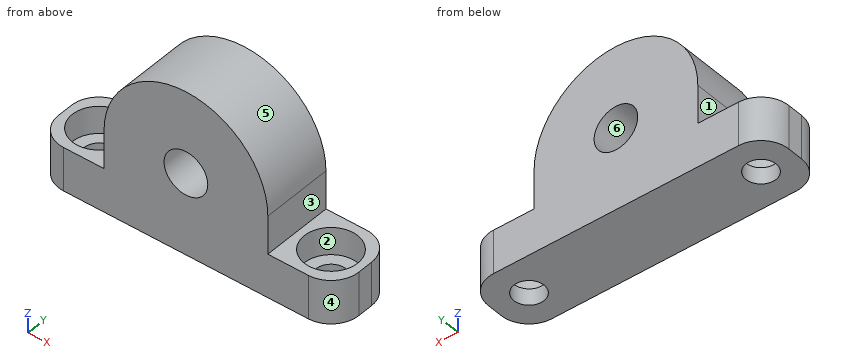
```python
from build123d import *

# Parameters (mm, degrees)
F0_R           = 4
F1_DEPTH       = 13
F3_D           = 5.5
F3_CBORE_D     = 9.75
F3_CBORE_DEPTH = 5
F4_R           = 5.08


with BuildPart() as f1:
    # F0 (on Front) → F1 (new body)
    with BuildSketch(Plane.XZ):
        with BuildLine():
            Line((-27.5, 8), (-27.5, 0))
            Line((-27.5, 0), (27.5, 0))
            Line((27.5, 0), (27.5, 8))
            Line((27.5, 8), (15, 8))
            Line((15, 8), (15, 15))
            ThreePointArc((15, 15), (0, 30), (-15, 15))
            Line((-15, 15), (-15, 8))
            Line((-15, 8), (-27.5, 8))
        make_face()
        with Locations((0, 15)):
            Circle(F0_R, mode=Mode.SUBTRACT)
    extrude(amount=F1_DEPTH)

    # F3 (through all)
    with Locations(Plane.XY.offset(8)):
        with Locations((-21.25, -6.5), (21.25, -6.5)):
            CounterBoreHole(F3_D / 2, F3_CBORE_D / 2, F3_CBORE_DEPTH)

    # F4
    f4_edges = [f1.edges().sort_by_distance(p)[0] for p in [
        (27.5, -13, 4),
        (27.5, 0, 4),
        (-27.5, -13, 4),
        (-27.5, 0, 4),
    ]]
    fillet(f4_edges, radius=F4_R)


solid = f1.part
```
Geometry: final body of the model. Coordinates: model frame, mm. Face numbers are marked on the shaded views. A direction names the side the tool comes from. Give positions to 0.01 mm unless a question says otherwise; leave off trailing zeros. Loops run counter-clockwise (first coordinate to the right, second up) from the corner with the lowest first, then second, coordinate; pieces in that order, holes last. Notation, with made-up numbers: (-11.75, 41) -> (28.25, 41) arc R21 ccw to (28.25, 69) -> close; hole circle Ø8 at (89.25, 38). An arc over 180 degrees is marked (long way). Return JSON: item names as keys, results as strings.
Item 1: Pin query (flat end, axial travel): P1, Ø4, axis at x = -16, y = -11, coming from the -Z side; P2, Ø3.5, axis at y = -9.5, z = 12.5, coming from the +X side; P3, Ø2, axis at x = -11.5, y = -7, coming from the +Z side; P4, Ø6, axis at x = -18.5, y = -5, coming from the +Z side. Return the tip coordinate at first contact, or that it passes through.
Filled in:
{"P1": "z = 0", "P2": "x = 15", "P3": "z = 25.71", "P4": "z = 8"}
Item 2: Line query: line 1 (Y direction, x = 21.25, z = 0.7); line 2 (Z direction, x = 0, y = -7); line 3 (Y direction, x = -21.25, z = 6.3) (3 decimals). Output: solid intervals per line, ascending.
Filled in:
{"line 1": "-13 to -9.25, -3.75 to 0", "line 2": "0 to 11, 19 to 30", "line 3": "-13 to -11.375, -1.625 to 0"}
Item 3: Section D-D, the plane y = -10.5. Output: boundary loops of the cut face in (x, z), plus the area to 3 significant figures.
Filled in:
{"outline": "(-26.8, 0) -> (26.8, 0) -> (26.8, 8) -> (24.04, 8) -> (24.04, 3) -> (18.46, 3) -> (18.46, 8) -> (15, 8) -> (15, 15) arc R15 ccw to (-15, 15) -> (-15, 8) -> (-18.46, 8) -> (-18.46, 3) -> (-24.04, 3) -> (-24.04, 8) -> (-26.8, 8) -> close; hole circle Ø8 at (0, 15)", "area": "886 mm^2"}
Item 4: Access query for the marked faces 1, 2 and 3. Directions: +Z, -Z, +X, -X, +Y, -Y. A direction counts if a zero-diameter tool reaches every point of the face in a straight line with its end or side. Return the directions, or none.
Filled in:
{"face 1": "+Z, -X, +Y, -Y", "face 2": "+Z", "face 3": "+Z, +X, +Y, -Y"}
Item 5: Mould query, pull axis Z, two halves, no side actions, for the marked faces 4, 5 and 6. Classes: released by +Z, released by -Z, zero draft, split by the parting line, or undercut.
Filled in:
{"face 4": "zero draft", "face 5": "released by +Z", "face 6": "undercut"}
Item 6: Section C-C, the plane z = 5. Output: boundary loops of the cut face in (x, y) (3 decimals), plus the area to 3 significant figures.
Filled in:
{"outline": "(-27.5, -7.92) arc R5.08 ccw to (-22.42, -13) -> (22.42, -13) arc R5.08 ccw to (27.5, -7.92) -> (27.5, -5.08) arc R5.08 ccw to (22.42, 0) -> (-22.42, 0) arc R5.08 ccw to (-27.5, -5.08) -> close; hole circle Ø9.75 at (-21.25, -6.5); hole circle Ø9.75 at (21.25, -6.5)", "area": "544 mm^2"}
Item 7: Section B-B, the plane x = 0. Output: boundary loops of the cut face in (y, z), plus the area to 3 significant figures.
Filled in:
{"outline": "(-13, 0) -> (0, 0) -> (0, 11) -> (-13, 11) -> close; (-13, 19) -> (0, 19) -> (0, 30) -> (-13, 30) -> close", "area": "286 mm^2"}
Item 8: Section A-A, the plane y = -6.5. Output: boundary loops of the cut face in (x, z) (3 decimals), plus the area to 3 significant figures.
Filled in:
{"outline": "(-27.5, 0) -> (-24, 0) -> (-24, 3) -> (-26.125, 3) -> (-26.125, 8) -> (-27.5, 8) -> close; (-18.5, 0) -> (18.5, 0) -> (18.5, 3) -> (16.375, 3) -> (16.375, 8) -> (15, 8) -> (15, 15) arc R15 ccw to (-15, 15) -> (-15, 8) -> (-16.375, 8) -> (-16.375, 3) -> (-18.5, 3) -> close; (24, 0) -> (27.5, 0) -> (27.5, 8) -> (26.125, 8) -> (26.125, 3) -> (24, 3) -> close; hole circle Ø8 at (0, 15)", "area": "823 mm^2"}
